Build history of the part. All positions in model axes, mm. A direction names the side the tool comes from. Round coordinates to 2 decimals unless told otherwise and drop trailing zeros. Write each loop counter-clockwise with the first axis right and the second up, starting at its lowest first coordinate (ties: lowest second). Pieces come first, ordered by that corner, then holes. Notation, with made-up numbers: (23.25, 23.25) -> (36.25, 23.25) arc R16 ccw to (36.25, 31.25) -> close; hole circle Ø6 at (55, 14.25). An arc over 180 degrees is marked (long way). One line per question, with ' | ' between items.
from build123d import *

# Parameters (mm, degrees)
EXTRUDE_1_DEPTH     = 5.33
SKETCH_1_W          = 0.5
SKETCH_1_H          = 0.5
EXTRUDE_2_DEPTH     = 2.54
SKETCH_1_2_W        = 0.5
SKETCH_1_2_H        = 0.5
EXTRUDE_3_DEPTH     = 10.16
SKETCH_4_R          = 0.2
CUT_EXTRUDE_1_DEPTH = 0.5
SKETCH_5_W          = 0.5
SKETCH_5_H          = 10.2
EXTRUDE_4_DEPTH     = 1.25
CUT_EXTRUDE_2_DEPTH = 1
FILLET_1_R          = 0.5
FILLET_2_R          = 1
SKETCH_7_W          = 0.5
SKETCH_7_H          = 0.5
CUT_EXTRUDE_3_DEPTH = 7.5
SKETCH_8_R          = 0.124451118
CUT_EXTRUDE_4_DEPTH = 1


with BuildPart() as part:
    # Sketch 3 → Extrude 1 (new body)
    with BuildSketch(Plane.XY.offset(2.54)):
        with BuildLine():
            Line((-0.325, -1.53), (3.105, -1.53))
            Line((3.105, -1.53), (3.99, 0))
            ThreePointArc((3.99, 0), (3.240904038, 1.868477631), (1.39, 2.66))
            ThreePointArc((1.39, 2.66), (-0.460904038, 1.868477631), (-1.21, 0))
            Line((-1.21, 0), (-0.325, -1.53))
        make_face()
    extrude(amount=EXTRUDE_1_DEPTH)

    # Sketch 1 → Extrude 2 (add)
    with BuildSketch(Plane.XY):
        with Locations((1.39, 0)):
            Rectangle(SKETCH_1_W, SKETCH_1_H)
        Rectangle(SKETCH_1_W, SKETCH_1_H)
        with Locations((2.78, 0)):
            Rectangle(SKETCH_1_W, SKETCH_1_H)
    extrude(amount=EXTRUDE_2_DEPTH)

    # Sketch 1_2 → Extrude 3 (add)
    with BuildSketch(Plane.XY):
        with Locations((1.39, 0)):
            Rectangle(SKETCH_1_2_W, SKETCH_1_2_H)
        Rectangle(SKETCH_1_2_W, SKETCH_1_2_H)
        with Locations((2.78, 0)):
            Rectangle(SKETCH_1_2_W, SKETCH_1_2_H)
    extrude(amount=-EXTRUDE_3_DEPTH)

    # Sketch 4 → Cut-Extrude 1 (cut)
    with BuildSketch(Plane.XY.offset(7.87)):
        with Locations(Location((2.78, 0, 0), (0, 0, 180))):
            Circle(SKETCH_4_R)
    extrude(amount=-CUT_EXTRUDE_1_DEPTH, mode=Mode.SUBTRACT)

    # Sketch 5 → Extrude 4 (add)
    with BuildSketch(Plane(origin=(0, -0.25, 0), x_dir=(1, 0, 0), z_dir=(0, 1, 0))):
        with Locations((1.39, 5.06)):
            Rectangle(SKETCH_5_W, SKETCH_5_H)
    extrude(amount=-EXTRUDE_4_DEPTH)

    # Sketch 6 → Cut-Extrude 2 (cut)
    with BuildSketch(Plane(origin=(1.64, 0, 0), x_dir=(0, 0, -1), z_dir=(1, 0, 0))):
        with BuildLine():
            Line((2.46, -1), (10.787068804, -1))
            Line((10.787068804, -1), (10.787068804, 0.83850211))
            Line((10.787068804, 0.83850211), (10.787068804, 2.125358058))
            Line((10.787068804, 2.125358058), (2.46, 2.125358058))
            Line((2.46, 2.125358058), (0.46, 2.125358058))
            Line((0.46, 2.125358058), (0.46, -0.5))
            ThreePointArc((0.46, -0.5), (0.606446609, -0.853553391), (0.96, -1))
            Line((0.96, -1), (2.46, -1))
        make_face()
    extrude(amount=-CUT_EXTRUDE_2_DEPTH, mode=Mode.SUBTRACT)

    # Fillet 1
    fillet_1_edges = [part.edges().sort_by_distance(p)[0] for p in [
        (1.39, -0.25, 0.04),
    ]]
    fillet(fillet_1_edges, radius=FILLET_1_R)

    # Fillet 2
    fillet_2_edges = [part.edges().sort_by_distance(p)[0] for p in [
        (1.39, -1.5, 0.04),
        (1.39, 0.25, -0.46),
    ]]
    fillet(fillet_2_edges, radius=FILLET_2_R)

    # Sketch 7 → Cut-Extrude 3 (cut)
    with BuildSketch(Plane(origin=(0, 0, -10.16), x_dir=(-1, 0, 0), z_dir=(0, 0, -1))):
        with Locations((-1.39, -1.25)):
            Rectangle(SKETCH_7_W, SKETCH_7_H)
        Rectangle(SKETCH_7_W, SKETCH_7_H)
        with Locations((-2.78, 0)):
            Rectangle(SKETCH_7_W, SKETCH_7_H)
    extrude(amount=-CUT_EXTRUDE_3_DEPTH, mode=Mode.SUBTRACT)

    # Sketch 8 → Cut-Extrude 4 (cut)
    with BuildSketch(Plane(origin=(0, 0, -2.66), x_dir=(-1, 0, 0), z_dir=(0, 0, -1))):
        with Locations((-1.39, -1.25)):
            Circle(SKETCH_8_R)
    extrude(amount=-CUT_EXTRUDE_4_DEPTH, mode=Mode.SUBTRACT)


solid = part.part
(1) Mould opens along X. For faces 3 (the flat face through (1, 1, 7.87)), 4 (the flat face through (1.14, -0.7, -0.2)), 5 (the flat face through (3.54, -0.78, 5.17)) say: pulls with the +X half, pulls with the -X half, needs draft (parallel to the pull), parting line crosses it, or undercut.
Calculated:
face 3: needs draft | face 4: undercut | face 5: pulls with the +X half
(2) 3-axis set-ups, long thin cutter, end or side, ignore diameter. For faces 1 (the flat face through (1.64, -0.7, -0.2)), 2 (the flat face through (-0.774, -0.754, 5.168)): which of +Z, -Z, +X, -X, +Y, -Y reach the whole face in a straight line?
Calculated:
face 1: -Z, +Y, -Y | face 2: +Z, -Z, -X, -Y
(3) Wall check: line 1 (Y direction, x = 0.1, z = -0.75); line 2 (Z direction, x = 2.7, y = 2.1); line 3 (Y direction, x = 2.78, z = 7.7). Give the ranges that are in metal, low to high. Write a range as from..to.
Calculated:
line 1: -0.25..0.25 | line 2: 2.54..7.87 | line 3: -1.53..-0.2, 0.2..2.24
(4) Slice it at D-D (y = 1.8). Write the cut outline in (x, z).
Calculated:
outline: (-0.53, 2.54) -> (3.31, 2.54) -> (3.31, 7.87) -> (-0.53, 7.87) -> close
(5) Slice it at B-B (x = 2.78). Write the cut outline in (y, z).
Calculated:
outline: (-1.53, 2.54) -> (-0.25, 2.54) -> (-0.25, -2.66) -> (0.25, -2.66) -> (0.25, 2.54) -> (2.24, 2.54) -> (2.24, 7.87) -> (0.2, 7.87) -> (0.2, 7.37) -> (-0.2, 7.37) -> (-0.2, 7.87) -> (-1.53, 7.87) -> close
(6) Drop flat-ended pins along their axis: pin 1 (1.3 mm diameter, centred on x = 0, y = 1, fed in from -Z); pin 2 (1 mm diameter, centred on y = 1, z = 2, fed in from -X); pin 3 (1.5 mm diameter, centred on y = 1, z = 6.5, fed in from +X); pin 4 (0.6 mm diameter, centred on y = 0, z = 0, fed in from +X). Give the stop position or say it passes through.
Calculated:
pin 1: z = 2.54 | pin 2: through | pin 3: x = 3.98 | pin 4: x = 3.03
(7) Slice it at C-C (z = 5.5). Write the cut outline in (x, y) (3 decimals).
Calculated:
outline: (-1.21, 0) -> (-0.325, -1.53) -> (3.105, -1.53) -> (3.99, 0) arc R2.63 ccw to (1.39, 2.66) arc R2.63 ccw to start
(8) Slice it at A-A (z = -1.25). Write the cut outline in (x, y).
Calculated:
outline: (-0.25, -0.25) -> (0.25, -0.25) -> (0.25, 0.25) -> (-0.25, 0.25) -> close; (1.14, -1.5) -> (1.64, -1.5) -> (1.64, -1) -> (1.14, -1) -> close; (2.53, -0.25) -> (3.03, -0.25) -> (3.03, 0.25) -> (2.53, 0.25) -> close
